Part model, mm, in its own coordinate system. A direction names the side the tool comes from. Round coordinates to 2 decimals unless told otherwise and drop trailing zeros. Loops run counter-clockwise (first coordinate to the right, second up) from the corner with the lowest first, then second, coordinate; pieces in that order, holes last. Notation, with made-up numbers: (22.25, 52.5) -> (48.25, 52.5) arc R18 cw to (48.25, 59.5) -> close; hole circle Ø9 at (10.25, -24). An arc over 180 degrees is marked (long way). Answer as CSV lines item,"result".
from build123d import *

# Parameters (mm, degrees)
SKETCH_R             = 1.9
PAD_DEPTH            = 5
SKETCH001_R          = 4
POCKET_DEPTH         = 3
FILLET_R             = 2
FILLET001_R          = 0.75
FILLET002_R          = 1.49
FILLET003_R          = 2.5
BODY_PLACEMENT_ANGLE = 270


with BuildPart() as part:
    # Sketch → Pad (new body)
    with BuildSketch(Plane.XZ):
        Polygon((4, 0), (-144.5, 0), (-144.5, -1.6), (-147.5, -1.6), (-147.5, 0), (-163.728138112, 0), (-163.728138112, -3.090405), (-169.728138112, -3.090405), (-169.728138112, 3.2), (-130.5, 3.2), (-130.5, 8.8), (-169.728138112, 8.8), (-169.728138112, 16.699631), (-163.728138112, 16.699631), (-163.728138112, 12), (-147.5, 12), (-147.5, 13.6), (-144.5, 13.6), (-144.5, 12), (4, 12), align=None)
        with Locations((-66, 6)):
            Circle(SKETCH_R, mode=Mode.SUBTRACT)
        with Locations((-6, 6)):
            Circle(SKETCH_R, mode=Mode.SUBTRACT)
        with Locations((-107.6, 6)):
            Circle(SKETCH_R, mode=Mode.SUBTRACT)
    extrude(amount=PAD_DEPTH)

    # Sketch001 (on Face24 of Pad) → Pocket (cut)
    with BuildSketch(Plane(origin=(0, 0, 0), x_dir=(1, 0, 0), z_dir=(0, 1, 0))):
        with Locations((-107.6, -6)):
            Circle(SKETCH001_R)
        with Locations((-66, -6)):
            Circle(SKETCH001_R)
        with Locations((-6, -6)):
            Circle(SKETCH001_R)
    extrude(amount=-POCKET_DEPTH, mode=Mode.SUBTRACT)

    # Fillet
    fillet_edges = [part.edges().sort_by_distance(p)[0] for p in [
        (4, -2.5, 12),
        (4, -2.5, 0),
    ]]
    fillet(fillet_edges, radius=FILLET_R)

    # Fillet001
    fillet001_edges = [part.edges().sort_by_distance(p)[0] for p in [
        (-147.5, -2.5, 12),
        (-147.5, -2.5, 13.6),
        (-144.5, -2.5, 13.6),
        (-144.5, -2.5, 12),
        (-144.5, -2.5, -1.6),
        (-147.5, -2.5, 0),
        (-147.5, -2.5, -1.6),
        (-144.5, -2.5, 0),
    ]]
    fillet(fillet001_edges, radius=FILLET001_R)

    # Fillet002
    fillet002_edges = [part.edges().sort_by_distance(p)[0] for p in [
        (-163.728138, -2.5, 0),
        (-163.728138, -2.5, -3.090405),
        (-169.728138, -2.5, -3.090405),
        (-169.728138, -2.5, 3.2),
        (-169.728138, -2.5, 16.699631),
        (-163.728138, -2.5, 16.699631),
        (-163.728138, -2.5, 12),
        (-169.728138, -2.5, 8.8),
    ]]
    fillet(fillet002_edges, radius=FILLET002_R)

    # Fillet003
    fillet003_edges = [part.edges().sort_by_distance(p)[0] for p in [
        (-130.5, -2.5, 8.8),
        (-130.5, -2.5, 3.2),
    ]]
    fillet(fillet003_edges, radius=FILLET003_R)


with BuildPart() as part_1:
    # Body placement: moved
    add(part.part.moved(Location((113, 136, 8))).rotate(Axis((113, 136, 8), (0, 0, -1)), BODY_PLACEMENT_ANGLE))


solid = part_1.part
Q1. Which spindle directions (+Z, -Z, +X, -X, +Y, -Y) get a long thin tool onto all of the face, cutting with end or side? Do faces 1 (the face through (115, -14, 16.8)), 2 (the face through (116, 29, 16)), 3 (the face through (115, -19, 20)). Say none if no direction does.
Geometry results:
face 1,"+X, -X, -Y"
face 2,"-X"
face 3,"+Z, +X, -X"
Q2. Saw through at B-B, the plane x = 116.85. Give the number of separate pieces and of enclosed holes in the cut face, then the cut area to 3 significant figures.
Geometry results:
separate pieces,"1"
enclosed holes,"3"
area,"1,890 mm2"
Q3. Drop flat-ended pins along their axis: P1, Ø1, axis at x = 116.5, y = 84.5, coming from the -Z side; P2, Ø0.5, axis at x = 115, y = -10, coming from the +Z side; P3, Ø1.5, axis at x = 116.5, y = 96.5, coming from the +Z side. Give the stop position or say it passes through.
Geometry results:
P1,"z = 8"
P2,"z = 21.6"
P3,"z = 20"
Q4. Saw through at C-C, the plane y = 130. Write the cut outline in (x, z).
Geometry results:
outline,"(113, 8) -> (118, 8) -> (118, 12.1) -> (116, 12.1) -> (116, 10) -> (113, 10) -> close; (113, 18) -> (116, 18) -> (116, 15.9) -> (118, 15.9) -> (118, 20) -> (113, 20) -> close"
Q5. Two-plate mould, pull along Y, no slides. Class faces 4 (the face through (114.479, 24.404, 13.824)), 5 (the face through (115, -33.728, 21)), 6 (the face through (113, 54, 13)): pulls with the +Y half, pulls with the -Y half, needs draft (parallel to the pull), parting line crosses it, or undercut.
Geometry results:
face 4,"undercut"
face 5,"pulls with the -Y half"
face 6,"needs draft"
Q6. Saw through at D-D, the plane y = 84.5. Write the cut outline in (x, z).
Geometry results:
outline,"(113, 8) -> (118, 8) -> (118, 20) -> (113, 20) -> close"
Q7. Drill centre lines: line 1 along Z through (x, y) = (117.4, 130); line 2 along Z through (x, y) = (114.85, 130); line 3 along Y through (x, z) = (117.4, 14). Where is each one in solid material? Low to high.
Geometry results:
line 1,"8 to 12.1, 15.9 to 20"
line 2,"8 to 10, 18 to 20"
line 3,"5.5 to 26.5, 30.3 to 68.1, 71.9 to 128.1, 131.9 to 140"
Q8. Saw through at A-A, the plane y = -15. Write the cut outline in (x, z), then the cut area to 3 significant figures.
Geometry results:
outline,"(113, 8) -> (118, 8) -> (118, 11.2) -> (113, 11.2) -> close; (113, 16.8) -> (118, 16.8) -> (118, 20) -> (113, 20) -> close"
area,"32.0 mm2"
